```python
from build123d import *

# Parameters (mm, degrees)
SKETCH001_W     = 13.272844
SKETCH001_H     = 19.997346
SKETCH001_W_2   = 7
SKETCH001_H_2   = 12
POCKET_DEPTH    = 11
SKETCH002_R     = 2.1
POCKET001_DEPTH = 53.501
SKETCH003_R     = 2.2
POCKET002_DEPTH = 77.001


with BuildPart() as part:
    # Sketch → Revolution (revolve)
    with BuildSketch(Plane.XZ):
        Polygon((0, 0), (50, 0), (50, 7), (27.4, 7), (9.4, 25), (7.4, 25), (7.4, 61), (4.9, 61), (4.9, 77), (0, 77), align=None)
    revolve(axis=Axis((0, 0, 0), (0, 0, 1)))

    # Sketch001 (on DatumPlane) → Pocket (cut)
    with BuildSketch(Plane(origin=(0, 0, 77), x_dir=(-1, 0, 0), z_dir=(0, 0, 1))):
        Rectangle(SKETCH001_W, SKETCH001_H)
        Rectangle(SKETCH001_W_2, SKETCH001_H_2, mode=Mode.SUBTRACT)
    extrude(amount=-POCKET_DEPTH, mode=Mode.SUBTRACT)

    # Sketch002 (on DatumPlane) → Pocket001 (cut, through all)
    with BuildSketch(Plane(origin=(3.5, 0, 0), x_dir=(0, 0, 1), z_dir=(1, 0, 0))):
        with Locations((72, 0)):
            Circle(SKETCH002_R)
    extrude(amount=-POCKET001_DEPTH, mode=Mode.SUBTRACT)

    # Sketch003 (on DatumPlane) → Pocket002 (cut, through all)
    with BuildSketch(Plane(origin=(0, 0, 0), x_dir=(1, 0, 0), z_dir=(0, 0, -1))):
        with Locations((30, 30)):
            Circle(SKETCH003_R)
        with Locations((-30, 30)):
            Circle(SKETCH003_R)
        with Locations((-30, -30)):
            Circle(SKETCH003_R)
        with Locations((30, -30)):
            Circle(SKETCH003_R)
    extrude(amount=-POCKET002_DEPTH, mode=Mode.SUBTRACT)


solid = part.part
```
Verification items for the finished model (mm, model axes). A direction names the side the tool comes from. Coordinates: 2 decimals unless noted, no trailing zeros. Loops run counter-clockwise (first coordinate to the right, second up) from the corner with the lowest first, then second, coordinate; pieces in that order, holes last. Notation, with made-up numbers: (-10.75, 18.5) -> (33.25, 18.5) arc R6 cw to (33.25, 27.5) -> close; hole circle Ø11 at (60.5, 12.5). An arc over 180 degrees is marked (long way). Put each result on its own line as item: value.
1. Section check B-B, the plane y = 30. Record the boundary of the cut face in (x, z), then the cut area to 3 significant figures.
Result set:
outline: (-40, 0) -> (-32.2, 0) -> (-32.2, 7) -> (-40, 7) -> close; (-27.8, 0) -> (27.8, 0) -> (27.8, 7) -> (-27.8, 7) -> close; (32.2, 0) -> (40, 0) -> (40, 7) -> (32.2, 7) -> close
area: 498 mm^2
2. Thickness scan on line 1 (X direction, y = -30, z = 1.75); line 2 (Z direction, x = 15.5, y = 26). Record the ranges inside material, lowest first.
Result set:
line 1: x = -40 to -32.2, -27.8 to 27.8, 32.2 to 40
line 2: z = 0 to 7
3. Section check D-D, the plane y = 0. Record the boundary of the cut face in (x, z).
Result set:
outline: (-50, 0) -> (50, 0) -> (50, 7) -> (27.4, 7) -> (9.4, 25) -> (7.4, 25) -> (7.4, 61) -> (4.9, 61) -> (4.9, 66) -> (3.5, 66) -> (3.5, 69.9) -> (-3.5, 69.9) -> (-3.5, 66) -> (-4.9, 66) -> (-4.9, 61) -> (-7.4, 61) -> (-7.4, 25) -> (-9.4, 25) -> (-27.4, 7) -> (-50, 7) -> close; (-3.5, 74.1) -> (3.5, 74.1) -> (3.5, 77) -> (-3.5, 77) -> close
4. Mould release check, pull along X, two halves, no side actions. Record for faces 4 (the face through (-1.604, -7.224, 43.252)), 5 (the face through (29.523, -27.852, 3.451)), 6 (the face through (29.523, 32.148, 3.451)), 7 (the face through (1, 1, 0)): pulls with the +X half, pulls with the -X half, needs draft (parallel to the pull), parting line crosses it, or undercut.
Result set:
face 4: parting line crosses it
face 5: undercut
face 6: undercut
face 7: needs draft
5. Gauge pin test, flat ends, axial feed: P1, Ø2, axis at y = -0.5, z = 73.5, coming from the -X side; P2, Ø6, axis at y = 5, z = 34.5, coming from the -X side; P3, Ø5, axis at x = 30, y = -30, coming from the -Z side; P4, Ø1.5, axis at x = -9, z = 8.5, coming from the -Y side. Record the tip position at first contact, or that the pin passes through.
Result set:
P1: stops at x = -3.5
P2: stops at x = -7.12
P3: stops at z = 0
P4: stops at y = -25.13
6. Section check A-A, the plane z = 72. Record the boundary of the cut face in (x, y), then the cut area to 3 significant figures.
Result set:
outline: (-3.5, -3.43) arc R4.9 ccw to (3.5, -3.43) -> (3.5, -2.1) -> (-3.5, -2.1) -> close; (-3.5, 2.1) -> (3.5, 2.1) -> (3.5, 3.43) arc R4.9 ccw to (-3.5, 3.43) -> close
area: 32.8 mm^2
7. Tool access check on faces 1 (the face through (-3.5, 2, 70)), 2 (the face through (5, -2, 61)), 3 (the face through (3.5, 2, 70)). Record the directions out of +Z, -Z, +X, -X, +Y, -Y that give a thin tool (end or side, any length) a straight path to the whole face; none if there is none.
Result set:
face 1: +Z, -X, +Y, -Y
face 2: +Z
face 3: +Z, +X, +Y, -Y
